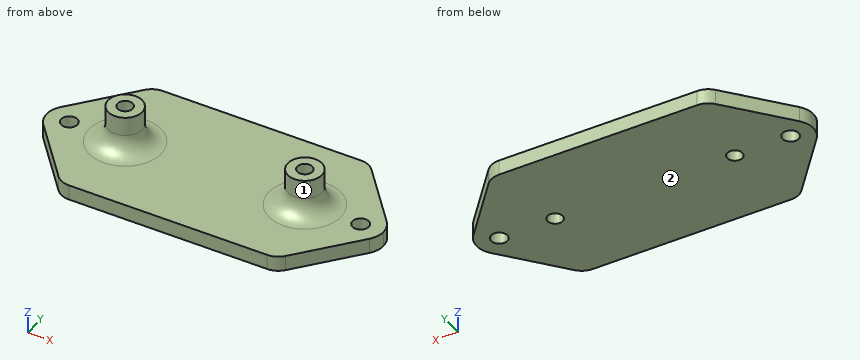
from build123d import *

# Parameters (mm, degrees)
F0_W     = 57
F0_H     = 42
F0_R     = 4.5
F0_R_2   = 2.15
F0_R_3   = 2
F1_DEPTH = 4
F2_DEPTH = 14
F3_R     = 5


with BuildPart() as f1:
    # F0 (on Top) → F1 (new body)
    with BuildSketch(Plane.XY):
        Rectangle(F0_W, F0_H)
        with Locations((-23.75, 0)):
            Circle(F0_R, mode=Mode.SUBTRACT)
        with Locations((23.75, 0)):
            Circle(F0_R, mode=Mode.SUBTRACT)
        with BuildLine():
            Line((-43.068388, -3.889709), (-28.5, -21))
            Line((-28.5, -21), (-28.5, 21))
            Line((-28.5, 21), (-43.068388, 3.889709))
            ThreePointArc((-43.068388, 3.889709), (-36.427601, 5.630734), (-32.5, 0))
            ThreePointArc((-32.5, 0), (-36.427601, -5.630734), (-43.068388, -3.889709))
        make_face()
        with BuildLine():
            Line((28.5, 21), (28.5, -21))
            Line((28.5, -21), (43.068388, -3.889709))
            ThreePointArc((43.068388, -3.889709), (32.5, 0), (43.068388, 3.889709))
            Line((43.068388, 3.889709), (28.5, 21))
        make_face()
        with BuildLine():
            ThreePointArc((-43.068388, 3.889709), (-44.5, 0), (-43.068388, -3.889709))
            ThreePointArc((-43.068388, -3.889709), (-36.427601, -5.630734), (-32.5, 0))
            ThreePointArc((-32.5, 0), (-36.427601, 5.630734), (-43.068388, 3.889709))
        make_face()
        with Locations((-38.5, 0)):
            Circle(F0_R_2, mode=Mode.SUBTRACT)
        with BuildLine():
            ThreePointArc((43.068388, 3.889709), (32.5, 0), (43.068388, -3.889709))
            ThreePointArc((43.068388, -3.889709), (44.130734, -2.072399), (44.5, 0))
            ThreePointArc((44.5, 0), (44.130734, 2.072399), (43.068388, 3.889709))
        make_face()
        with Locations((38.5, 0)):
            Circle(F0_R_2, mode=Mode.SUBTRACT)
        with Locations((-23.75, 0)):
            Circle(F0_R)
        with Locations((-23.75, 0)):
            Circle(F0_R_3, mode=Mode.SUBTRACT)
        with Locations((23.75, 0)):
            Circle(F0_R)
        with Locations((23.75, 0)):
            Circle(F0_R_3, mode=Mode.SUBTRACT)
    extrude(amount=F1_DEPTH)

    # F0 (on Top) → F2 (join)
    with BuildSketch(Plane.XY):
        with Locations((-23.75, 0)):
            Circle(F0_R)
        with Locations((-23.75, 0)):
            Circle(F0_R_3, mode=Mode.SUBTRACT)
        with Locations((23.75, 0)):
            Circle(F0_R)
        with Locations((23.75, 0)):
            Circle(F0_R_3, mode=Mode.SUBTRACT)
    extrude(amount=F2_DEPTH)

    # F3
    f3_edges = [f1.edges().sort_by_distance(p)[0] for p in [
        (-28.5, 21, 2),
        (-28.5, -21, 2),
        (28.5, -21, 2),
        (28.5, 21, 2),
        (-28.25, 0, 4),
        (19.25, 0, 4),
    ]]
    fillet(f3_edges, radius=F3_R)


solid = f1.part
Here's how the part is built. I have some questions about the finished solid (model axes, mm). Face numbers are marked on the shaded views. Coordinates: 2 decimals unless noted, no trailing zeros. Write each loop counter-clockwise with the first axis right and the second up, starting at its lowest first coordinate (ties: lowest second). Pieces come first, ordered by that corner, then holes.
Item 1: I want a section at A-A on x = -23.75. Write out the boundary of the cut face in (y, z), and give its area (3 significant figures).
Item 2: I want a section at B-B on z = 10.75. Write out the boundary of the cut face in (x, y), and give its area (3 significant figures).
Item 3: I want a section at C-C on x = 7. Write out the boundary of the cut face in (y, z).
Item 4: Will these pins go through, and if not, where does the flat tip stop? pin 1 (3 mm diameter, centred on x = -23.75, y = 0, fed in from -Z); pin 2 (8 mm diameter, centred on y = 4, z = 12, fed in from -X); pin 3 (3 mm diameter, centred on x = -13.5, y = -7, fed in from +Z); pin 4 (1 mm diameter, centred on x = -31, z = 1.5, fed in from +Y).
Item 5: If we mould it in two halves opening along X, with no side actions, what happens to the marked faces 1 and 2? For each: +X half, -X half, draft (parallel to the pull), parting line (faces both ways), or undercut.
Item 6: I want a section at D-D on x = 38.5. Write out the boundary of the cut face in (y, z), and give its area (3 significant figures).
Item 7: If I drill on line 1 (Y direction, x = 23.75, z = 3.5); line 2 (Z direction, x = -36.5, y = -2); line 3 (X direction, y = -1, z = 12.5), over which ranges is the centre line in solid material (lowest first)?
Findings below:
1. outline: (-21, 0) - (-2, 0) - (-2, 14) - (-4.5, 14) - (-4.5, 9) arc R5 cw to (-9.5, 4) - (-21, 4) - close; (2, 0) - (21, 0) - (21, 4) - (9.5, 4) arc R5 cw to (4.5, 9) - (4.5, 14) - (2, 14) - close
1. area: 213 mm2
2. outline: circle Ø9 at (-23.75, 0); circle Ø9 at (23.75, 0); hole circle Ø4 at (-23.75, 0); hole circle Ø4 at (23.75, 0)
2. area: 102 mm2
3. outline: (-21, 0) - (21, 0) - (21, 4) - (-21, 4) - close
4. pin 1: passes through
4. pin 2: stops at x = -28.25
4. pin 3: stops at z = 4
4. pin 4: stops at y = 18.65
5. face 1: undercut
5. face 2: draft
6. outline: (-9.26, 0) - (-2.15, 0) - (-2.15, 4) - (-9.26, 4) - close; (2.15, 0) - (9.26, 0) - (9.26, 4) - (2.15, 4) - close
6. area: 56.8 mm2
7. line 1: y = -21 to -2, 2 to 21
7. line 2: z = 0 to 4
7. line 3: x = -28.14 to -25.48, -22.02 to -19.36, 19.36 to 22.02, 25.48 to 28.14
